For this review, take the finished solid that the model builds, in its own axes (mm). A direction names the side the tool comes from. Round coordinates to 2 decimals unless told otherwise and drop trailing zeros. Loops run counter-clockwise (first coordinate to the right, second up) from the corner with the lowest first, then second, coordinate; pieces in that order, holes last. Notation, with made-up numbers: (68.5, -39) -> (110.5, -39) arc R18 ccw to (110.5, -27) -> close; hole circle Ø8 at (51, 40). An arc over 180 degrees is marked (long way). Use one line per item in the form item = value. Start each with the question number.
from build123d import *

# Parameters (mm, degrees)
F1_DEPTH = 5


with BuildPart() as f1:
    # F0 (on Top) → F1 (new body)
    with BuildSketch(Plane.XY):
        with BuildLine():
            Line((26.669694, 11.429262), (-52.970227, 11.429262))
            ThreePointArc((-52.970227, 11.429262), (-63.433421, -0.472084), (-50.289965, -9.324771))
            Line((-50.289965, -9.324771), (26.031774, -9.324771))
            Line((26.031774, -9.324771), (26.063537, -8.29138))
            ThreePointArc((26.063537, -8.29138), (23.106773, 1.66914), (26.669694, 11.429262))
        make_face()
        with BuildLine():
            ThreePointArc((56.184654, 0.453414), (45.418068, 16.673179), (26.669694, 11.429262))
            ThreePointArc((26.669694, 11.429262), (23.106773, 1.66914), (26.063537, -8.29138))
            ThreePointArc((26.063537, -8.29138), (39.001798, -15.377065), (52.454503, -9.324771))
            Line((52.454503, -9.324771), (45.693033, -9.324771))
            ThreePointArc((45.693033, -9.324771), (43.571713, -8.446092), (42.693033, -6.324771))
            Line((42.693033, -6.324771), (42.693033, -2.546586))
            ThreePointArc((42.693033, -2.546586), (43.571713, -0.425266), (45.693033, 0.453414))
            Line((45.693033, 0.453414), (56.184654, 0.453414))
        make_face()
    extrude(amount=F1_DEPTH)


solid = f1.part
Item 1: Take a section at A-A on z = 3.7. Give the boundary of the cut face in (x, y).
Item 2: For P1, Ø4, axis at x = -13, y = -11, coming from the +Z side; P2, Ø3, axis at x = -45, z = 3.5, coming from the -Y side; P3, Ø2.5, axis at x = 50.5, z = 3, coming from the +Y side, all flat-tipped, find the tip position at first contact; note any pin that passes through.
Item 3: Take a section at B-B on x = -19. Give the boundary of the cut face in (y, z).
Item 4: Take a section at C-C on y = -5. Give the boundary of the cut face in (x, z), plus the area to 3 significant figures.
Item 5: Wall thickness on line 1 (Y direction, x = 6, z = 2.8); line 2 (X direction, y = 1.5, z = 1.3); line 3 (X direction, y = -12.5, z = 1.7): over which ranges is each line inside the solid? List them lowest first.
Item 6: Machinability: for faces 1 (the flat face through (51, 0.453, 2)), 2 (the flat face through (-4, 1, 0)), 3 (the flat face through (-13, 11.429, 2)), which of the approach directions +Z, -Z, +X, -X, +Y, -Y give a long, thin tool a straight path to every point of the face, cutting with its end or side? Answer none if there is none.
Item 7: Draft analysis for pull direction Y (two halves, no side actions). For faces 4 (the cylindrical face through (43.595, -8.469, 2.465)), 5 (the flat face through (-13, -9.325, 2)), 6 (the flat face through (-4, 1, 5)), state which applies: +Y half, -Y half, draft (parallel to the pull), parting line (faces both ways), or undercut.
Results:
q1.outline = (-52.97, 11.43) arc R10.55 ccw (long way) to (-50.29, -9.32) -> (26.03, -9.32) -> (26.06, -8.29) arc R16.55 ccw to (52.45, -9.32) -> (45.69, -9.32) arc R3 cw to (42.69, -6.32) -> (42.69, -2.55) arc R3 cw to (45.69, 0.45) -> (56.18, 0.45) arc R16.55 ccw to (26.67, 11.43) -> close
q2.P1 = 5
q2.P2 = -9.32
q2.P3 = 14.64
q3.outline = (-9.32, 0) -> (11.43, 0) -> (11.43, 5) -> (-9.32, 5) -> close
q4.outline = (-61.73, 0) -> (42.69, 0) -> (42.69, 5) -> (-61.73, 5) -> close
q4.area = 522 mm2
q5.line_1 = -9.32 to 11.43
q5.line_2 = -63.5 to 56.2
q5.line_3 = 30.31 to 48.99
q6.face_1 = +Z, -Z, +X
q6.face_2 = -Z, +X, -X, +Y, -Y
q6.face_3 = +Z, -Z, -X, +Y
q7.face_4 = undercut
q7.face_5 = -Y half
q7.face_6 = draft
